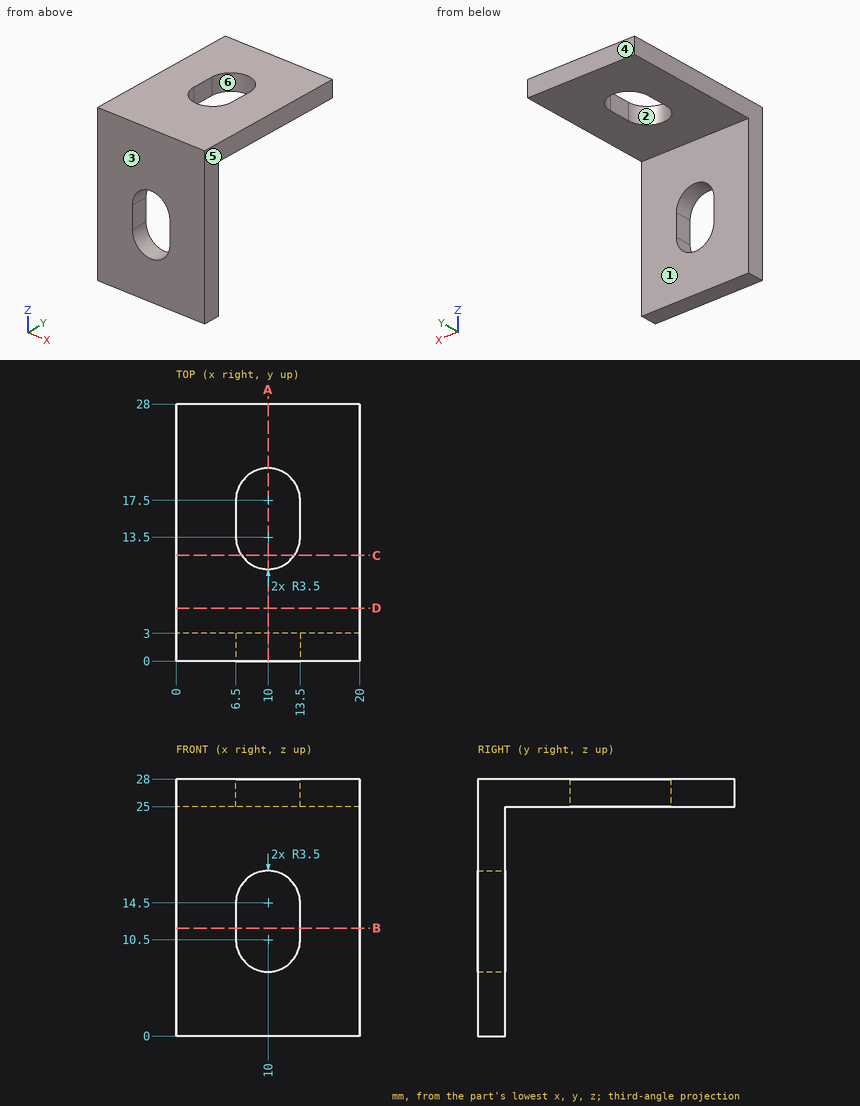
Study the drawing (mm; zero at the part's minimum x, y, z) and answer. A direction names the side the tool comes from. Coordinates: 2 decimals unless noted, no trailing zeros. Write each loop counter-clockwise with the first axis right and the second up, starting at its lowest first coordinate (ties: lowest second). Pieces come first, ordered by that corner, then holes. Notation, with made-up numbers: (76.5, 83) - (115.5, 83) arc R8 ccw to (115.5, 97) - close; hole circle Ø2 at (1.25, 59). An arc over 180 degrees is marked (long way). Answer as a JSON object with one key per item and string values.
Q1. For a pull along Y with two mould halves and no side action, classify the marked faces 4, 5 and 6 as pulls with the +Y half, pulls with the -Y half, needs draft (parallel to the pull), parting line crosses it, or undercut.
Results list:
{"face 4": "pulls with the +Y half", "face 5": "needs draft", "face 6": "undercut"}
Q2. Find section B-B (z = 11.75). Write down the section's boundary in (x, y).
Results list:
{"outline": "(0, 0) - (6.5, 0) - (6.5, 3) - (0, 3) - close; (13.5, 0) - (20, 0) - (20, 3) - (13.5, 3) - close"}
Q3. Find section C-C (y = 11.5). Write down the section's boundary in (x, z), plus the area to 3 significant figures.
Results list:
{"outline": "(0, 25) - (7.13, 25) - (7.13, 28) - (0, 28) - close; (12.87, 25) - (20, 25) - (20, 28) - (12.87, 28) - close", "area": "42.8 mm^2"}
Q4. Given pin 1 Ø6 at (y, z) = (5.5, 3.5) entering from -X; pin 2 Ø6 at (x, y) = (15, 16) entering from -Z, each flat-ended and moving along its own axis, determine where each tip first touches the part or whether it passes through.
Results list:
{"pin 1": "stops at x = 0", "pin 2": "stops at z = 25"}
Q5. Which of the six approach directions +Z, -Z, +X, -X, +Y, -Y give full straight-line access (tool end or side, diameter ignored) to the marked faces 1, 2 and 3?
Results list:
{"face 1": "-Z, +X, -X, +Y", "face 2": "+Z, -Z", "face 3": "+Z, -Z, +X, -X, -Y"}
Q6. Find section D-D (y = 5.75). Write down the section's boundary in (x, z), plus the area to 3 significant figures.
Results list:
{"outline": "(0, 25) - (20, 25) - (20, 28) - (0, 28) - close", "area": "60.0 mm^2"}
Q7. Find section A-A (x = 10). Write down the section's boundary in (y, z), plus the area to 3 significant figures.
Results list:
{"outline": "(0, 0) - (3, 0) - (3, 7) - (0, 7) - close; (0, 18) - (3, 18) - (3, 25) - (10, 25) - (10, 28) - (0, 28) - close; (21, 25) - (28, 25) - (28, 28) - (21, 28) - close", "area": "93.0 mm^2"}
Q8. Consider L1, parallel to Z at x = 18, y = 25.5; L2, parallel to Y at x = 3, z = 22.25; L3, parallel to X at y = 2.5, z = 15. Determine where each line is inside the solid, lowest interval first. Write a range as from..to.
Results list:
{"L1": "z = 25..28", "L2": "y = 0..3", "L3": "x = 0..6.54, 13.46..20"}
